Here's how the part is built. I have some questions about the finished solid (model axes, mm). A direction names the side the tool comes from. Coordinates: 2 decimals unless noted, no trailing zeros. Loops run counter-clockwise (first coordinate to the right, second up) from the corner with the lowest first, then second, coordinate; pieces in that order, holes last. Notation, with made-up numbers: M 23.5,4.25 L 75.5,4.25 A31 cw 75.5,32.25 Z; hole C 33,-25 d1. An arc over 180 degrees is marked long. Use CSV: the item, a comma, the result in double quotes. Start each with the question number.
Q1. If we section it at B-B (x = 0): State how many separate pieces and enclosed holes the cut face has, and give its area (3 significant figures).
Q2. If we section it at C-C (z = 18.5): Please give me the cut outline in (x, y).
Q3. Please list where these lines run through material, in increasing order: probe 1 along Y at (x, z) = (0, -24.35); probe 2 along X at (y, z) = (60, -21); probe 3 along Z at (x, y) = (-3, 58). Write a range as [from, to].
Q4. If we section it at A-A (y = 70.5): Please give me the cut outline in (x, z).
Q5. If we mould it in two halves opening along Y, with no side actions, what happens to faces 1 (the flat face through (-12.7, 54, -22)), 2 (the cylindrical face through (11.917, 10.208, 0.553)), 3 (the flat face through (-11.3, 88.9, -2))? For each: +Y half, -Y half, draft (parallel to the pull), parting line (faces both ways), or undercut.
Q6. Which directions (+Z, -Z, +X, -X, +Y, -Y) give clear straight access to the entire face, cutting with the end or side of a thin tool? Please do faces 4 (the flat face through (-11.112, 71, 0)), 5 (the cylindrical face through (-11.895, 73.935, 11.522)).
from build123d import *

# Parameters (mm, degrees)
SKETCH1_W              = 25.4
SKETCH1_H              = 50.8
SKETCH1_W_2            = 22.225
SKETCH1_H_2            = 47.625
EXTRUDE_THIN1_DEPTH    = 88.9
F_10_CLEARANCE_HOLE1_D = 5.1054
F_10_CLEARANCE_HOLE2_D = 5.1054
SKETCH8_R              = 23.8125
CUT_EXTRUDE1_DEPTH     = 26.4


with BuildPart() as part:
    # Sketch1 → Extrude-Thin1 (new body)
    with BuildSketch(Plane(origin=(0, 0, 0), x_dir=(1, 0, 0), z_dir=(0, 1, 0))):
        Rectangle(SKETCH1_W, SKETCH1_H)
        Rectangle(SKETCH1_W_2, SKETCH1_H_2, mode=Mode.SUBTRACT)
    extrude(amount=EXTRUDE_THIN1_DEPTH)

    # #10 Clearance Hole1 (through all)
    with Locations(Plane.ZY.offset(12.7)):
        with Locations((-12.7, 76.2), (0, 76.2), (12.7, 76.2), (-12.7, 12.7), (0, 12.7), (12.7, 12.7)):
            Hole(F_10_CLEARANCE_HOLE1_D / 2)

    # #10 Clearance Hole2 (through all)
    with Locations(Plane.XY.offset(25.4)):
        with Locations((0, 12.7), (0, 76.2), (0, 44.45)):
            Hole(F_10_CLEARANCE_HOLE2_D / 2)

    # Sketch8 → Cut-Extrude1 (cut, through all)
    with BuildSketch(Plane.ZY.offset(12.7)):
        with Locations((0, 44.45)):
            Circle(SKETCH8_R)
    extrude(amount=-CUT_EXTRUDE1_DEPTH, mode=Mode.SUBTRACT)


solid = part.part
Results below:
1,separate pieces,"8"
1,enclosed holes,"0"
1,area,"234 mm^2"
2,outline,"M -12.7,0 L -11.11,0 L -11.11,29.46 L -12.7,29.46 Z; M -12.7,59.44 L -11.11,59.44 L -11.11,88.9 L -12.7,88.9 Z; M 11.11,0 L 12.7,0 L 12.7,29.46 L 11.11,29.46 Z; M 11.11,59.44 L 12.7,59.44 L 12.7,88.9 L 11.11,88.9 Z"
3,probe 1,"[0, 10.15], [15.25, 41.9], [47, 73.65], [78.75, 88.9]"
3,probe 2,"[-12.7, -11.11], [11.11, 12.7]"
3,probe 3,"[-25.4, -23.81], [23.81, 25.4]"
4,outline,"M -12.7,-25.4 L 12.7,-25.4 L 12.7,25.4 L -12.7,25.4 Z; hole M -11.11,-23.81 L 11.11,-23.81 L 11.11,23.81 L -11.11,23.81 Z"
5,face 1,"draft"
5,face 2,"undercut"
5,face 3,"+Y half"
6,face 4,"+Y, -Y"
6,face 5,"+X, -X"
